Here's how the part is built. I have some questions about the finished solid (model axes, mm). A direction names the side the tool comes from. Coordinates: 2 decimals unless noted, no trailing zeros. Write each loop counter-clockwise with the first axis right and the second up, starting at its lowest first coordinate (ties: lowest second). Pieces come first, ordered by that corner, then holes. Notation, with made-up numbers: (73.25, -19) - (87.25, -19) arc R26 ccw to (87.25, 17) - close; hole circle Ø5 at (-12, 81.25). An arc over 180 degrees is marked (long way). Answer in a Markdown table with one row per item. Add a question column.
Item 1: We'd pull the mould along Y, two halves only. Please class faces 3 (the face through (-28, -49, 2)), 4 (the face through (30, -10, 2)), 5 (the face through (26.996, -28.538, 2.465)): +Y half, -Y half, draft (parallel to the pull), parting line (faces both ways), or undercut.
Item 2: Imagine slicing it at C-C (y = -27.5). Please give me the cut outline in (x, z), plus the area to 3 significant figures.
Item 3: Imagine slicing it at B-B (x = 0). Please give me the cut outline in (y, z), plus the area to 3 significant figures.
Item 4: Imagine slicing it at A-A (y = -10). Please give me the cut outline in (x, z), plus the area to 3 significant figures.
Item 5: Imagine slicing it at D-D (x = -24). Please give me the cut outline in (y, z).
Item 6: I'm going to push flat-ended pins straight in: pin 1 (1.2 mm diameter, centred on x = -11.5, y = -31, fed in from +Z); pin 2 (2.5 mm diameter, centred on x = -25, y = -45, fed in from +Z). Where does each tip first touch, or does it pass through?
Item 7: Which directions (+Z, -Z, +X, -X, +Y, -Y) give clear straight access to the entire face, cutting with the end or side of a thin tool? Please do faces 1 (the face through (25.2, -9.73, 2.97)), 2 (the face through (-23.631, -43.214, 2.465)).
Item 8: If I drill on probe 1 along X at (y, z) = (25, 2.85); probe 2 along Y at (x, z) = (25, 2.85); probe 3 along Y at (x, z) = (-24, 4.55), over which ranges is the centre line in solid material (lowest first)? Write a range as from..to.
Autodesk Inventor part; units mm, degrees
ref_plane "YZ Plane" through (0, 0, 0) normal (1, 0, 0) x (0, 1, 0)
ref_plane "XZ Plane" through (0, 0, 0) normal (0, 1, 0) x (-1, 0, 0)
ref_plane "XY Plane" through (0, 0, 0) normal (0, 0, 1) x (1, 0, 0)
sketch "Sketch2" plane through (0, 0, 0) normal (0, 0, 1) x (1, 0, 0)
  line L0 (-25, -50) -> (25, -50)
  arc A0 (25, -50) -> (30, -45) centre (25, -45) ccw
  line L1 (30, -45) -> (30, 25)
  arc A1 (30, 25) -> (25, 30) centre (25, 25) ccw
  line L2 (25, 30) -> (-25, 30)
  arc A2 (-25, 30) -> (-30, 25) centre (-25, 25) ccw
  line L3 (-30, 25) -> (-30, -45)
  arc A3 (-30, -45) -> (-25, -50) centre (-25, -45) ccw
  circle A4 centre (25, -27.5) radius 1.621
  circle A5 centre (-25, 7.5) radius 1.621
  circle A6 centre (-25, -27.5) radius 1.621
  circle A7 centre (25, 7.5) radius 1.621
  line L4 (20, 16) -> (20, -36)
  arc A8 (16, -40) -> (20, -36) centre (16, -36) ccw
  line L5 (16, -40) -> (-16, -40)
  arc A9 (-20, -36) -> (-16, -40) centre (-16, -36) ccw
  line L6 (-20, -36) -> (-20, 16)
  arc A10 (-16, 20) -> (-20, 16) centre (-16, 16) ccw
  line L7 (-16, 20) -> (16, 20)
  arc A11 (20, 16) -> (16, 20) centre (16, 16) ccw
  circle A12 centre (25, 25) radius 1.621
  circle A13 centre (-25, -45) radius 1.621
  circle A14 centre (25, -45) radius 1.621
  circle A15 centre (-25, 25) radius 1.621
  point P0 (0, 0)
extrude "Extrusion1" add sketch "Sketch2" along normal blind 5 contours A3 L3 A2 L2 A1 L1 A0 L0 | L4 A8 L5 A9 L6 A10 L7 A11
sketch "Sketch3" plane through (0, 0, 5) normal (0, 0, 1) x (1, 0, 0)
  circle A0 centre (0, -10) radius 15
  line L0 (25, 30) -> (-25, 30) construction
  arc A1 (-25, 30) -> (-30, 25) centre (-25, 25) ccw construction
  line L1 (-30, 25) -> (-30, -45) construction
  arc A2 (-30, -45) -> (-25, -50) centre (-25, -45) ccw construction
  line L2 (-25, -50) -> (25, -50) construction
  arc A3 (25, -50) -> (30, -45) centre (25, -45) ccw construction
  line L3 (30, -45) -> (30, 25) construction
  arc A4 (30, 25) -> (25, 30) centre (25, 25) ccw construction
  line L4 (-25, -45) -> (25, 25) construction
  line L5 (25, -45) -> (-25, 25) construction
  dimension "d6" = 30
extrude "Extrusion2" cut sketch "Sketch3" against normal blind 5
sketch "Sketch6" plane through (0, 0, 5) normal (0, 0, 1) x (1, 0, 0)
  line L0 (30, -45) -> (30, 25) construction
  line L1 (25, 30) -> (-25, 30) construction
  line L2 (-30, 25) -> (-30, -45) construction
  line L3 (-25, -50) -> (25, -50) construction
  line L4 (16, -40) -> (-16, -40) construction
  line L5 (-20, -36) -> (-20, 16) construction
  line L6 (-16, 20) -> (16, 20) construction
  line L7 (20, 16) -> (20, -36) construction
  circle A0 centre (25, -27.5) radius 1.621 construction
  circle A1 centre (-25, 7.5) radius 1.621 construction
  circle A2 centre (-25, 25) radius 1.621 construction
  circle A3 centre (25, -45) radius 1.621 construction
  circle A4 centre (-25, -45) radius 1.621 construction
  circle A5 centre (25, 25) radius 1.621 construction
  circle A6 centre (-25, -27.5) radius 1.621 construction
  circle A7 centre (25, 7.5) radius 1.621 construction
  arc A8 (-30, -45) -> (-25, -50) centre (-25, -45) ccw
  arc A9 (25, -50) -> (30, -45) centre (25, -45) ccw
  arc A10 (30, 25) -> (25, 30) centre (25, 25) ccw
  arc A11 (-25, 30) -> (-30, 25) centre (-25, 25) ccw
  arc A12 (-20, -36) -> (-16, -40) centre (-16, -36) ccw
  arc A13 (-16, 20) -> (-20, 16) centre (-16, 16) ccw
  arc A14 (20, 16) -> (16, 20) centre (16, 16) ccw
  arc A15 (16, -40) -> (20, -36) centre (16, -36) ccw
hole "Hole3" at (-25, -45, 5) at (-25, -27.5, 5) at (-25, 7.5, 5) at (-25, 25, 5) at (25, 25, 5) at (25, 7.5, 5) at (25, -27.5, 5) at (25, -45, 5) direction (0, 0, -1) diameter 4.5 end through all
sketch "Sketch7" plane through (0, 0, 5) normal (0, 0, 1) x (1, 0, 0)
  circle A0 centre (0, -10) radius 26.5 construction
  circle A1 centre (0, -10) radius 21.5 construction
  circle A2 centre (0, -10) radius 24 construction
  circle A3 centre (0, -10) radius 15 construction
  line L0 (-58.8, 0) -> (58.8, 0) construction
  line L1 (42, -10) -> (-42, -10) construction
  point P0 (-24, -10)
  point P1 (-12, -30.7846)
  point P2 (12, -30.7846)
  point P3 (24, -10)
  point P4 (12, 10.7846)
  point P5 (-12, 10.7846)
  dimension "d43" = 48
  dimension "d41" = 53
  dimension "d42" = 43
  dimension "d46" = 360
hole "Hole4" at (-24, -10, 5) at (-12, -30.7846, 5) at (12, -30.7846, 5) at (24, -10, 5) at (12, 10.7846, 5) at (-12, 10.7846, 5) direction (0, 0, -1) diameter 2.459 depth 4
equation "\"d43\" = 0.5 * d41 + 0.5 * d42"
properties part number "P017" material "Aluminium"
Here are the results:
| question | item | result |
|---|---|---|
| 1 | face 3 | -Y half |
| 1 | face 4 | draft |
| 1 | face 5 | undercut |
| 2 | outline | (-30, 0) - (-27.25, 0) - (-27.25, 5) - (-30, 5) - close; (-22.75, 0) - (22.75, 0) - (22.75, 5) - (-22.75, 5) - close; (27.25, 0) - (30, 0) - (30, 5) - (27.25, 5) - close |
| 2 | area | 255 mm2 |
| 3 | outline | (-50, 0) - (-25, 0) - (-25, 5) - (-50, 5) - close; (5, 0) - (30, 0) - (30, 5) - (5, 5) - close |
| 3 | area | 250 mm2 |
| 4 | outline | (-30, 0) - (-15, 0) - (-15, 5) - (-22.77, 5) - (-22.77, 1) - (-25.23, 1) - (-25.23, 5) - (-30, 5) - close; (15, 0) - (30, 0) - (30, 5) - (25.23, 5) - (25.23, 1) - (22.77, 1) - (22.77, 5) - (15, 5) - close |
| 4 | area | 130 mm2 |
| 5 | outline | (-50, 0) - (-47.02, 0) - (-47.02, 5) - (-50, 5) - close; (-42.98, 0) - (-29.52, 0) - (-29.52, 5) - (-42.98, 5) - close; (-25.48, 0) - (5.48, 0) - (5.48, 5) - (-8.77, 5) - (-8.77, 1) - (-11.23, 1) - (-11.23, 5) - (-25.48, 5) - close; (9.52, 0) - (22.98, 0) - (22.98, 5) - (9.52, 5) - close; (27.02, 0) - (30, 0) - (30, 5) - (27.02, 5) - close |
| 6 | pin 1 | stops at z = 1 |
| 6 | pin 2 | passes through |
| 7 | face 1 | +Z |
| 7 | face 2 | +Z, -Z |
| 8 | probe 1 | x = -30..-27.25, -22.75..22.75, 27.25..30 |
| 8 | probe 2 | y = -50..-47.25, -42.75..-29.75, -25.25..-10.72, -9.28..5.25, 9.75..22.75, 27.25..30 |
| 8 | probe 3 | y = -50..-47.02, -42.98..-29.52, -25.48..-11.23, -8.77..5.48, 9.52..22.98, 27.02..30 |
